Source: CAD feature listing. Evaluate the final solid. Frame: model axes, mm. Face numbers are marked on the shaded views. A direction names the side the tool comes from. Round coordinates to 2 decimals unless told otherwise and drop trailing zeros. Loops run counter-clockwise (first coordinate to the right, second up) from the corner with the lowest first, then second, coordinate; pieces in that order, holes last. Notation, with made-up numbers: M -20,29.5 L -5,29.5 A11 ccw -5,35.5 Z; hole C 50,-32 d9. An arc over 180 degrees is marked long. Write each question's results on one line, items separated by ' | '. Start each with the question number.
1. Contact query for flat-ended pins moving along their axis: pin 1 Ø1.5 at (x, z) = (-4.5, 4) entering from -Y; pin 2 Ø3 at (y, z) = (-3, 4.5) entering from -X; pin 3 Ø3 at (x, y) = (-0.5, 0) entering from +Z. Output: stop coordinate, or through.
2. Ray query, line 1 (Z direction, x = 10.5, y = -1); line 2 (Y direction, x = 0, z = 6); line 3 (Z direction, x = 9.5, y = -1.5). Return the intervals inside material, ascending.
3. Draft query along Y for the marked faces 3, 4 and 5. Return one class per face: released by +Y, released by -Y, zero draft, split by the parting line, or undercut.
4. Set-up query: the marked faces 1 and 2. Return all of +Z, -Z, +X, -X, +Y, -Y with unobstructed straight access to the full face (end or side cutting, diameter ignored); none if empty.
5. Section A-A on z = 4.5. Output: boundary loops of the cut face in (x, y), and give its area (3 significant figures).
6. Section C-C on x = -23. Output: boundary loops of the cut face in (y, z), and give its area (3 significant figures).
7. Section B-B on y = -12. Output: boundary loops of the cut face in (x, z).
8. Section D-D on z = -0.5. Output: boundary loops of the cut face in (x, y).
from build123d import *

# Parameters (mm, degrees)
F0_W     = 16
F0_H     = 1.2547565785
F3_R     = 1.725
F4_DEPTH = 7.3
F5_DEPTH = 3.5
F3_R_2   = 3
F6_DEPTH = 1


with BuildPart() as f1:
    # F0 (on Front) → F1 (revolve)
    with BuildSketch(Plane.XZ):
        Polygon((-7.7905750729, 7.2604851217), (-7.7905750729, 0), (8.2094249271, 0), (11.2094249271, 0), (11.2094249271, 3.4629283439), (9.7094249271, 3.4629283439), (9.7094249271, 5.4733994966), (8.2094249271, 5.4733994966), (8.2094249271, 7.2604851217), align=None)
        with Locations((0.2094249271, -0.6273782892)):
            Rectangle(F0_W, F0_H)
    revolve(axis=Axis((-7.7905750729, 0, 2.7390308408), (0, 0, 1)))

    # F3 (on offset) → F4 (cut)
    with BuildSketch(Plane.XY.offset(7.2604851217)):
        with Locations((-0.0100255911, 0.0691023806)):
            Circle(F3_R)
    extrude(amount=-F4_DEPTH, mode=Mode.SUBTRACT)

    # F3 (on offset) → F5 (cut)
    with BuildSketch(Plane.XY.offset(7.2604851217)):
        Polygon((-1.3136138991, 2.2415214753), (-2.5980214903, -0.0168622697), (-1.2844075912, -2.258383745), (1.3136138991, -2.2415214753), (2.5980214903, 0.0168622697), (1.2844075912, 2.258383745), align=None)
        with Locations((-0.0100255911, 0.0691023806)):
            Circle(F3_R, mode=Mode.SUBTRACT)
    extrude(amount=-F5_DEPTH, mode=Mode.SUBTRACT)

    # F3 (on offset) → F6 (cut)
    with BuildSketch(Plane.XY.offset(7.2604851217)):
        with Locations((-0.0100255911, 0.0691023806)):
            Circle(F3_R_2)
        Polygon((-1.2844075912, -2.258383745), (-2.5980214903, -0.0168622697), (-1.3136138991, 2.2415214753), (1.2844075912, 2.258383745), (2.5980214903, 0.0168622697), (1.3136138991, -2.2415214753), align=None, mode=Mode.SUBTRACT)
    extrude(amount=-F6_DEPTH, mode=Mode.SUBTRACT)


solid = f1.part
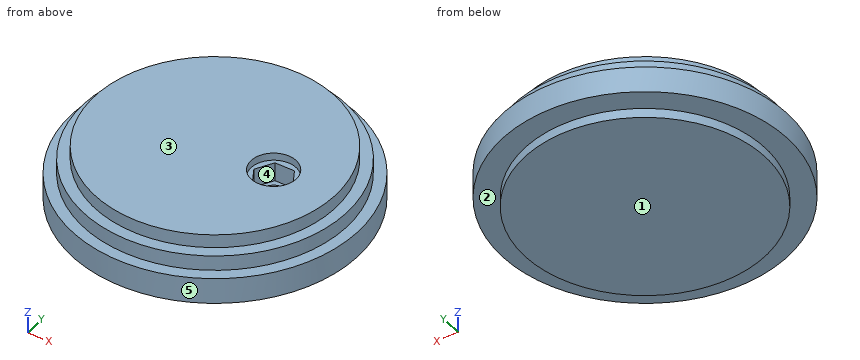
Taken from the geometry:
1) pin 1: y = -18.8 | pin 2: x = -26.69 | pin 3: z = 3.76
2) line 1: 0 to 3.46 | line 2: -13.98 to -2.25, 2.25 to 13.98 | line 3: 0 to 5.47
3) face 3: zero draft | face 4: undercut | face 5: split by the parting line
4) face 1: -Z, +X, -X, +Y, -Y | face 2: -Z
5) outline: C -7.79,0 d35; hole M -2.6,-0.02 L -1.28,-2.26 L 1.31,-2.24 L 2.6,0.02 L 1.28,2.26 L -1.31,2.24 Z | area: 945 mm^2
6) outline: M -11.39,0 L -4.97,0 L -4.97,-1.25 L 4.97,-1.25 L 4.97,0 L 11.39,0 L 11.39,3.46 L 8.66,3.46 L 8.66,5.47 L 4.97,5.47 L 4.97,7.26 L -4.97,7.26 L -4.97,5.47 L -8.66,5.47 L -8.66,3.46 L -11.39,3.46 Z | area: 144 mm^2
7) outline: M -22.52,0 L -18.37,0 L -18.37,-1.25 L 2.79,-1.25 L 2.79,0 L 6.94,0 L 6.94,3.46 L 4.95,3.46 L 4.95,5.47 L 2.79,5.47 L 2.79,7.26 L -18.37,7.26 L -18.37,5.47 L -20.53,5.47 L -20.53,3.46 L -22.52,3.46 Z
8) outline: C -7.79,0 d32
